Design review of the part built by this model. Coordinates are the model's own, in mm. A direction names the side the tool comes from. Round coordinates to 2 decimals unless told otherwise and drop trailing zeros. Write each loop counter-clockwise with the first axis right and the second up, starting at its lowest first coordinate (ties: lowest second). Pieces come first, ordered by that corner, then holes. Notation, with made-up numbers: (0.5, 34) -> (23.5, 34) arc R4 ccw to (23.5, 40) -> close; hole circle Ø9 at (14.25, -1). An arc over 180 degrees is marked (long way). Write item = value, one per line. Start each with the question number.
Item 1: Add section C-C, the plane x = 5. State the section outline as (y, z) points (3 decimals), then the cut area to 3 significant figures.
Item 2: For pin 1 Ø1.6 at (x, z) = (29.5, -0.5) entering from +Y; pin 2 Ø1.6 at (y, z) = (-38, 0.5) entering from +X; pin 3 Ø1.9 at (x, y) = (-40, 0) entering from +Z, all flat-tipped, find the tip position at first contact; note any pin that passes through.
Item 3: To check wall thickness, follow L1, parallel to Y at x = 41.75, z = 0; L2, parallel to X at y = 53.75, z = 0; L3, parallel to Z at x = -20, y = -56. State the ranges of each line that lie inside material, in increasing order.
Item 4: Add section B-B, the plane z = 3. State the section outline as (x, y) points (1 decimal), then the cut area to 3 significant figures.
Item 5: Add section A-A, the plane y = -23.36. State the section outline as (x, z) points (3 decimals).
Item 6: Add section D-D, the plane y = 0. State the section outline as (x, z) points.
Item 7: Mouldability with a two-part tool opening along Z and no side actions: class faces 6 (the flat face through (-1, 1, 5)), 7 (the flat face through (30, 52.5, 0)), 8 (the flat face through (45, 1, -2)) as released by +Z, released by -Z, zero draft, split by the parting line, or undercut.
Item 8: Machinability: for faces 1 (the flat face through (-1, 1, -5)), 2 (the flat face through (40, 0, 0)), 3 (the cylindrical face through (6.964, -8.403, -0.07)), 4 (the flat face through (30, -52.5, 0)), 5 (the flat face through (-40, 0, 0)), which of the approach directions +Z, -Z, +X, -X, +Y, -Y give a long, thin tool a straight path to every point of the face, cutting with its end or side? Answer none if there is none.
Autodesk Inventor part; units mm, degrees
ref_plane "YZ Plane" through (0, 0, 0) normal (1, 0, 0) x (0, 1, 0)
ref_plane "XZ Plane" through (0, 0, 0) normal (0, 1, 0) x (-1, 0, 0)
ref_plane "XY Plane" through (0, 0, 0) normal (0, 0, 1) x (1, 0, 0)
sketch "Sketch1" plane through (0, 0, 0) normal (0, 0, 1) x (1, 0, 0)
  line L0 (-45, 57.5) -> (45, 57.5)
  line L1 (45, 57.5) -> (45, -57.5)
  line L2 (45, -57.5) -> (-45, -57.5)
  line L3 (-45, -57.5) -> (-45, 57.5)
  line L4 (-45, 57.5) -> (45, -57.5) construction
  line L5 (45, 57.5) -> (-45, -57.5) construction
  point P0 (0, 0)
  dimension "d0" = 90
  dimension "d1" = 115
extrude "Extrusion1" add sketch "Sketch1" along normal mid plane 10
sketch "Sketch2" plane through (45, -57.5, 5) normal (1, 0, 0) x (0, 0, -1)
  line L0 (10, 0) -> (0, 0)
  line L1 (10, 115) -> (10, 0)
  point P0 (5, 57.5)
  point P1 (5, 20)
  point P2 (5, 57.5)
  point P3 (5, 95)
  dimension "d4" = 20
  dimension "d5" = 5
  dimension "d8" = 37.5
hole "Hole1" at (45, -37.5, 0) at (45, 0, 0) at (45, 37.5, 0) direction (-1, 0, 0) diameter 3.175 depth 5
sketch "Sketch3" plane through (-45, -57.5, 5) normal (0, -1, 0) x (1, 0, 0)
  line L0 (0, 0) -> (0, -10)
  line L1 (90, -10) -> (0, -10)
  point P0 (45, -5)
  point P1 (25, -5)
  point P2 (75, -5)
  dimension "d20" = 25
  dimension "d21" = 5
  dimension "d24" = 50
hole "Hole2" at (-20, -57.5, 0) at (30, -57.5, 0) direction (0, 1, 0) diameter 3.175 depth 5
sketch "Sketch4" plane through (-45, 57.5, 5) normal (0, 1, 0) x (1, 0, 0)
  line L0 (0, 10) -> (0, 0)
  line L1 (90, 0) -> (0, 0)
  point P0 (45, 5)
  point P1 (25, 5)
  point P2 (75, 5)
  dimension "d36" = 25
  dimension "d37" = 5
  dimension "d40" = 50
hole "Hole3" at (-20, 57.5, 0) at (30, 57.5, 0) direction (0, -1, 0) diameter 3.175 depth 5
sketch "Sketch5" plane through (0, 0, 5) normal (0, 0, 1) x (1, 0, 0)
  line L0 (-45, 57.5) -> (-45, -57.5)
  line L1 (-45, -57.5) -> (45, -57.5)
  point P0 (0, 0)
  point P1 (-40, -37.5)
  point P2 (-40, 0)
  point P3 (-40, 37.5)
  dimension "d52" = 5
  dimension "d53" = 20
  dimension "d56" = 37.5
hole "Hole4" at (-40, -37.5, 5) at (-40, 0, 5) at (-40, 37.5, 5) direction (0, 0, -1) diameter 3.175 depth 5
sketch "Sketch7" plane through (0, 0, -5) normal (0, 0, -1) x (-1, 0, 0)
  circle A0 centre (-5, -23.36) radius 15.085
  line L0 (-45, -57.5) -> (45, -57.5)
  line L1 (-45, 57.5) -> (-45, -57.5)
  point P0 (0, 0)
  dimension "d74" = 34.14
  dimension "d75" = 40
  dimension "d76" = 30.17
extrude "Extrusion3" cut sketch "Sketch7" against normal through all
thread "Thread1"
properties part number "left"
Result set:
q1.outline = (-57.5, -5) -> (-38.445, -5) -> (-38.445, 5) -> (-57.5, 5) -> close; (-8.275, -5) -> (57.5, -5) -> (57.5, 5) -> (-8.275, 5) -> close
q1.area = 848 mm²
q2.pin_1 = 52.5
q2.pin_2 = 40
q2.pin_3 = 0
q3.L1 = -57.5 to -39.09, -35.91 to -1.59, 1.59 to 35.91, 39.09 to 57.5
q3.L2 = -45 to -21.59, -18.41 to 28.41, 31.59 to 45
q3.L3 = -5 to -1.59, 1.59 to 5
q4.outline = (-45, -57.5) -> (45, -57.5) -> (45, 57.5) -> (-45, 57.5) -> close; hole circle Ø3.2 at (-40, -37.5); hole circle Ø3.2 at (-40, 0); hole circle Ø3.2 at (-40, 37.5); hole circle Ø30.2 at (5, -23.4)
q4.area = 9,610 mm²
q5.outline = (-45, -5) -> (-10.085, -5) -> (-10.085, 5) -> (-45, 5) -> close; (20.085, -5) -> (45, -5) -> (45, 5) -> (20.085, 5) -> close
q6.outline = (-45, -5) -> (45, -5) -> (45, -1.59) -> (40, -1.59) -> (40, 1.59) -> (45, 1.59) -> (45, 5) -> (-38.41, 5) -> (-38.41, 0) -> (-41.59, 0) -> (-41.59, 5) -> (-45, 5) -> close
q7.face_6 = released by +Z
q7.face_7 = undercut
q7.face_8 = zero draft
q8.face_1 = -Z, +X, -X, +Y, -Y
q8.face_2 = +X
q8.face_3 = +Z, -Z
q8.face_4 = -Y
q8.face_5 = +Z
